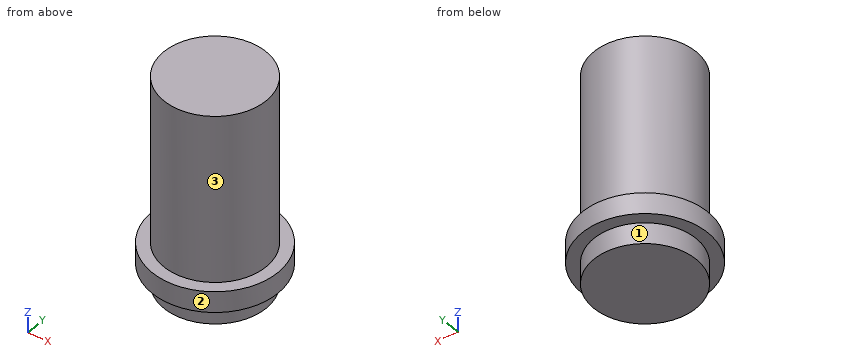
```python
from build123d import *

# Parameters (mm, degrees)
F0_R     = 4.875
F1_DEPTH = 20
F2_START = 2
F0_R_2   = 6
F2_DEPTH = 2


with BuildPart() as f1:
    # F0 (on Top) → F1 (new body)
    with BuildSketch(Plane.XY):
        Circle(F0_R)
    extrude(amount=F1_DEPTH)

    # F0 (on Top) → F2 (join)
    with BuildSketch(Plane.XY.offset(F2_START)):
        Circle(F0_R_2)
        Circle(F0_R, mode=Mode.SUBTRACT)
    extrude(amount=F2_DEPTH)


solid = f1.part
```
Check sheet for the modelled part. Datum: model origin and axes. Units: mm. Face numbers are marked on the shaded views. A direction names the side the tool comes from. Coordinates: 2 decimals unless noted, no trailing zeros. Order: outer loops, then holes, each group sorted by start corner. A loop starts at its lowest first (then second) coordinate and runs counter-clockwise, first axis right, second up. Notation, with made-up numbers: (6, -2.75) -> (37, -2.75) arc R9 ccw to (37, 1.25) -> close; hole circle Ø7 at (10, -9.5). An arc over 180 degrees is marked (long way). Write item = value, one per line. Start each with the question number.
1) Material ranges on L1, parallel to Z at x = -5.5, y = 1.25; L2, parallel to X at y = 1, z = 13.5; L3, parallel to Y at x = -4.25, z = 12.5, recorded low to high.
2) Access from +Z, -Z, +X, -X, +Y, -Y to the whole of each face (thin tool, end or side, straight path). Record for the marked faces 1, 2 and 3.
3) Cross-section at D-D (z = 3). Enter the section's corners in (x, y), then the cut area to 3 significant figures.
4) Cross-section at C-C (z = 7). Enter the section's corners in (x, y) (3 decimals).
5) Cross-section at A-A (x = 0). Enter the section's corners in (y, z) (3 decimals).
6) Go/stop test with flat-tipped pins: P1, Ø5, axis at x = 3.5, z = 2.5, coming from the +Y side; P2, Ø2, axis at y = 1, z = 9, coming from the +X side (3 decimals); P3, Ø4, axis at y = -2.5, z = 5.5, coming from the -X side. Record where each tip stops, or that it passes through.
Ans:
q1.L1 = 2 to 4
q1.L2 = -4.77 to 4.77
q1.L3 = -2.39 to 2.39
q2.face_1 = -Z
q2.face_2 = +Z, -Z
q2.face_3 = +Z
q3.outline = circle Ø12 at (0, 0)
q3.area = 113 mm²
q4.outline = circle Ø9.75 at (0, 0)
q5.outline = (-6, 2) -> (-4.875, 2) -> (-4.875, 0) -> (4.875, 0) -> (4.875, 2) -> (6, 2) -> (6, 4) -> (4.875, 4) -> (4.875, 20) -> (-4.875, 20) -> (-4.875, 4) -> (-6, 4) -> close
q6.P1 = 5.92
q6.P2 = 4.875
q6.P3 = -5.88
